The drawing under review shows one solid part. Ordinate dimensions are in mm from its lowest x, y, z. Coordinates: 2 decimals unless noted, no trailing zeros. Order: outer loops, then holes, each group sorted by start corner. A loop starts at its lowest first (then second) coordinate and runs counter-clockwise, first axis right, second up. Notation, with made-up numbers: M 63,74.25 L 95,74.25 A5 ccw 95,78.25 Z; hole C -26.75,-24 d6. An arc over 180 degrees is marked long. Answer as a JSON object with one key per item and string values.
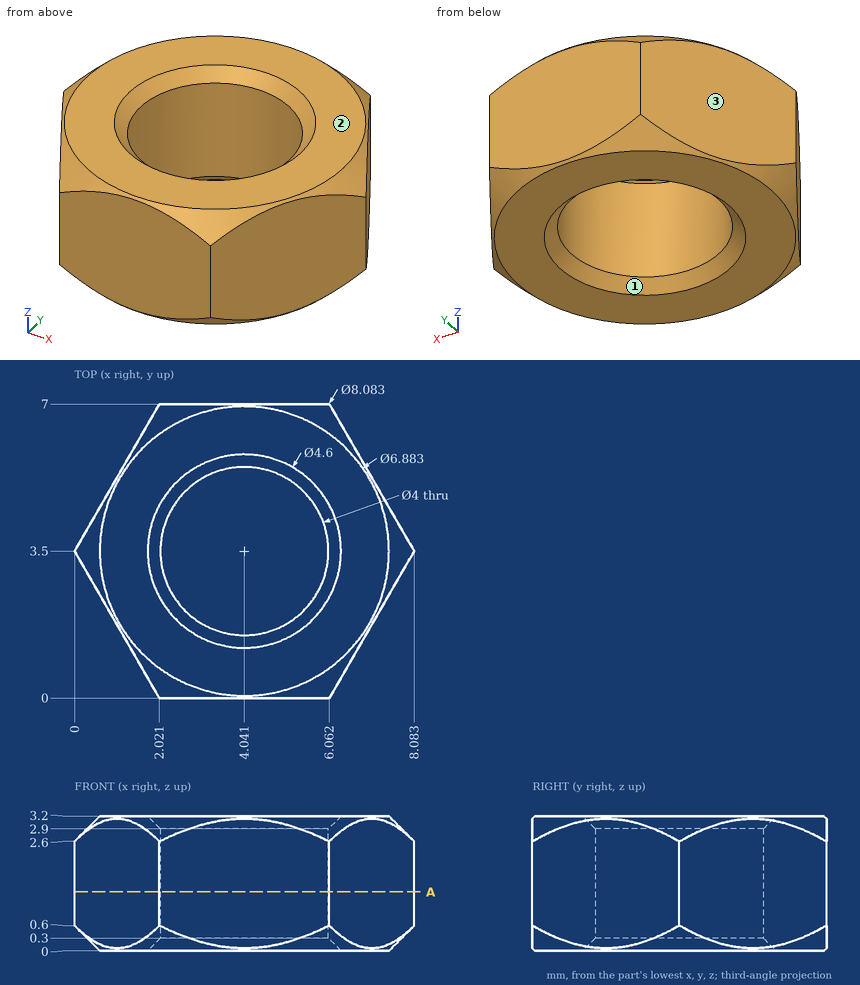
1) Mouldability with a two-part tool opening along Y and no side actions: class the marked faces 1, 2 and 3 as released by +Y, released by -Y, zero draft, split by the parting line, or undercut.
Taken from the geometry:
{"face 1": "undercut", "face 2": "zero draft", "face 3": "released by +Y"}
2) To check wall thickness, follow L1, parallel to Y at x = 3.75, z = 0.35; L2, parallel to X at y = 2.25, z = 1.05 (1 decimal); L3, parallel to X at y = 4, z = 2.15 (1 decimal). State the ranges of each line that lie inside material, in increasing order.
Taken from the geometry:
{"L1": "y = 0 to 1.52, 5.48 to 7", "L2": "x = 0.7 to 2.5, 5.6 to 7.4", "L3": "x = 0.3 to 2.1, 6 to 7.8"}
3) Add section A-A (z = 1.4). State the section outline as (x, y) points.
Taken from the geometry:
{"outline": "M 0,3.5 L 2.02,0 L 6.06,0 L 8.08,3.5 L 6.06,7 L 2.02,7 Z; hole C 4.04,3.5 d4"}
4) Insertion check: pin 1 Ø1 at (x, y) = (6.5, 4.5) entering from -Z. The pin has a flat end and moves straight along its axis. Give the tip position at first contact, or say it passes through.
Taken from the geometry:
{"pin 1": "stops at z = 0"}
